from build123d import *

# Parameters (mm, degrees)
SKETCH1_R           = 34.075
BOSS_EXTRUDE1_DEPTH = 50
FILLET1_R           = 34
SKETCH3_R           = 5.5
CUT_EXTRUDE1_DEPTH  = 57
BOSS_EXTRUDE2_DEPTH = 54
FILLET2_R           = 5
SKETCH5_R           = 28.2539
CUT_EXTRUDE2_DEPTH  = 27


with BuildPart() as part:
    # Sketch1 → Boss-Extrude1 (new body)
    with BuildSketch(Plane.XY):
        Circle(SKETCH1_R)
    extrude(amount=BOSS_EXTRUDE1_DEPTH)

    # Fillet1
    fillet1_edges = [part.edges().sort_by_distance(p)[0] for p in [
        (-34.075, 0, 50),
    ]]
    fillet(fillet1_edges, radius=FILLET1_R)

    # Sketch3 → Cut-Extrude1 (cut)
    with BuildSketch(Plane(origin=(0, 0, 0), x_dir=(-1, 0, 0), z_dir=(0, 0, -1))):
        with Locations((-11.427232, 12.850521)):
            Circle(SKETCH3_R)
        with Locations((9.257377, 12.850521)):
            Circle(SKETCH3_R)
    extrude(amount=-CUT_EXTRUDE1_DEPTH, mode=Mode.SUBTRACT)

    # Sketch4 → Boss-Extrude2 (add)
    with BuildSketch(Plane(origin=(0, 0, 0), x_dir=(-1, 0, 0), z_dir=(0, 0, -1))):
        with BuildLine():
            Line((-19.721396, -9.77574), (19.555863, -8.501695))
            ThreePointArc((19.555863, -8.501695), (0.554256, -28.777347), (-19.721396, -9.77574))
        make_face()
    extrude(amount=-BOSS_EXTRUDE2_DEPTH)

    # Fillet2
    fillet2_edges = [part.edges().sort_by_distance(p)[0] for p in [
        (-0.554256, -28.777347, 54),
        (0.082767, -9.138717, 54),
    ]]
    fillet(fillet2_edges, radius=FILLET2_R)

    # Sketch5 → Cut-Extrude2 (cut)
    with BuildSketch(Plane(origin=(0, 0, 0), x_dir=(-1, 0, 0), z_dir=(0, 0, -1))):
        Circle(SKETCH5_R)
    extrude(amount=-CUT_EXTRUDE2_DEPTH, mode=Mode.SUBTRACT)


solid = part.part
Can you work these out from the model? Positions are in its coordinate system, mm. A direction names the side the tool comes from. Coordinates: 2 decimals unless noted, no trailing zeros. Loops run counter-clockwise (first coordinate to the right, second up) from the corner with the lowest first, then second, coordinate; pieces in that order, holes last. Notation, with made-up numbers: (12.25, 47.25) - (57.25, 47.25) arc R18 ccw to (57.25, 75.25) - close; hole circle Ø7 at (9, -6.5). An arc over 180 degrees is marked (long way). Answer as a JSON object with one key per item and string values. Group by question number.
Item 1: For pin 1 (12 mm diameter, centred on x = 22.5, z = 5.5, fed in from -Y); pin 2 (1 mm diameter, centred on x = 11, y = -5, fed in from -Z); pin 3 (4 mm diameter, centred on x = -8.5, z = 8.5, fed in from -Y), each with a flat end and sliding along its axis, tell me the tip position at first contact or that it passes through.
Item 2: If we mould it in two halves opening along X, with no side actions, what happens to faces 1 (the face through (-26.95, 8.49, 13.31)), 2 (the face through (0, -19, 54)), 3 (the face through (-0.99, -28.76, 43.14))? For each: released by +X, released by -X, zero draft, split by the parting line, or undercut.
Item 3: On a 3-axis mill with a long thin cutter (end or side, diameter ignored), from which of +Z, -Z, +X, -X, +Y, -Y can I reach the whole of each face in a straight line? I mean faces 4 (the face through (8.89, 7.97, 35)), 5 (the face through (0, 0, 27)). Say none if no direction works.
Item 4: If I drill on L1, parallel to X at y = 1, z = 11; L2, parallel to Y at x = 0, z = 14 (3 decimals); L3, parallel to X at y = 16, z = 34, over which ranges is the centre line in solid material (lowest first)? Write a range as from..to.
Item 5: If we section it at A-A (z = 4): List the corners of the cut face in (x, y) for me (3 decimals), plus the area to 3 significant figures.
Returned:
{
 "1": {"pin 1": "stops at y = -29.81", "pin 2": "stops at z = 27", "pin 3": "stops at y = -33.45"},
 "2": {"face 1": "undercut", "face 2": "zero draft", "face 3": "split by the parting line"},
 "3": {"face 4": "+Z, -Z", "face 5": "-Z"},
 "4": {"L1": "x = -34.06..-28.24, 28.24..34.06", "L2": "y = -34.075..-28.254, 28.254..34.075", "L3": "x = -24.09..-13.77, -4.75..6.92, 15.94..24.09"},
 "5": {"outline": "circle Ø68.15 at (0, 0); hole circle Ø56.508 at (0, 0)", "area": "1,140 mm²"}
}
